Source: three-view drawing plus pictorial views. Frame: mm from the lowest corner of the part. A direction names the side the tool comes from. Give positions to 0.01 mm unless a question says otherwise; leave off trailing zeros. Write each loop counter-clockwise with the first axis right and the second up, starting at its lowest first coordinate (ties: lowest second). Pieces come first, ordered by that corner, then holes.
Q1. Cut plane D-D on x = 38. Return the cut outline in (y, z).
Q2. Pin query (flat end, axial travel): pin 1 (10 mm diameter, centred on x = 59, y = 28.5, fed in from +Z); pin 2 (2.5 mm diameter, centred on x = 42, z = 15, fed in from +Y); pin 3 (10 mm diameter, centred on y = 41.5, z = 6.5, fed in from -X); pin 4 (1.5 mm diameter, centred on y = 10.5, z = 6.5, fed in from -X). Return the tip coordinate at first contact, or that it passes through.
Q3. Cut plane A-A on y = 36.5. Return the cut outline in (x, z) (1 decimal), plus the area to 3 significant figures.
Q4. Reachability of the marked faces 1, 2 and 3 from +Z, -Z, +X, -X, +Y, -Y: full face, straight path, thin tool, end or side. Return the list, or none.
Q5. Cut plane B-B on x = 19.5. Return the cut outline in (y, z).
Q6. Line query: L1, parallel to Y at x = 33, z = 3.75; L2, parallel to Z at x = 48, y = 38; L3, parallel to X at y = 14, z = 16.5 (1 decimal). Output: solid intervals per line, ascending.
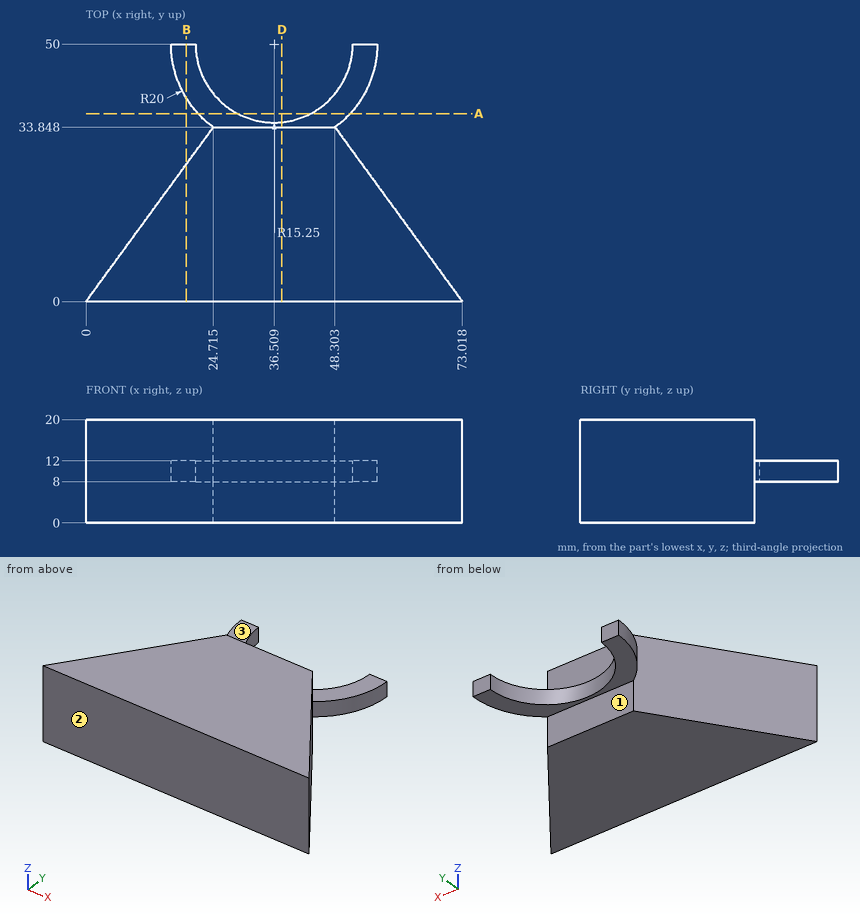
Data:
1. outline: (0, 0) - (33.85, 0) - (33.85, 8) - (34.82, 8) - (34.82, 12) - (33.85, 12) - (33.85, 20) - (0, 20) - close
2. pin 1: passes through
2. pin 2: stops at y = 33.85
2. pin 3: stops at x = 16.86
2. pin 4: stops at x = 7.12
3. outline: (21.8, 8) - (29.4, 8) - (29.4, 12) - (21.8, 12) - close; (43.6, 8) - (51.3, 8) - (51.3, 12) - (43.6, 12) - close
3. area: 61.3 mm2
4. face 1: -Z, +X, -X, +Y
4. face 2: +Z, -Z, +X, -X, -Y
4. face 3: +Z, +X, -X, +Y
5. outline: (0, 0) - (26.71, 0) - (26.71, 20) - (0, 20) - close; (39.48, 8) - (50, 8) - (50, 12) - (39.48, 12) - close
6. L1: y = 0 to 33.85
6. L2: z = 8 to 12
6. L3: x = 10.2 to 62.8
